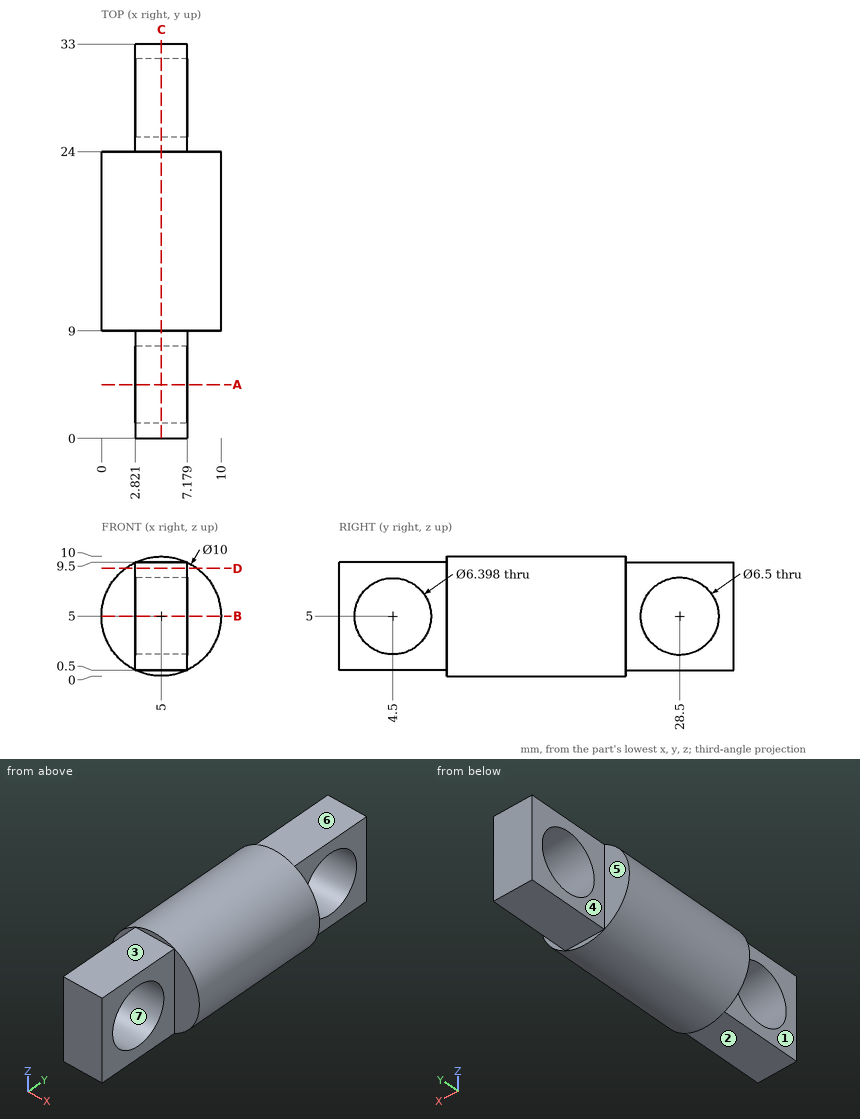
Can you work these out from the drawing? Everything is in mm from the part's minimum corner. A direction names the side the tool comes from. Give positions to 0.01 mm unless a question says otherwise; leave off trailing zeros. Order: outer loops, then holes, each group sorted by start corner. A loop starts at its lowest first (then second) coordinate and runs counter-clockwise, first axis right, second up. Notation, with made-up numbers: M 42.25,-8 L 46.25,-8 A9 cw 46.25,1 Z; hole C 62.5,-4 d4. An arc over 180 degrees is marked long. One line per item, written item: value.
Item 1: If we section it at A-A on y = 4.5: Write out the boundary of the cut face in (x, z).
Verdict:
outline: M 2.82,0.5 L 7.18,0.5 L 7.18,1.8 L 2.82,1.8 Z; M 2.82,8.2 L 7.18,8.2 L 7.18,9.5 L 2.82,9.5 Z
Item 2: For pin 1 (3 mm diameter, centred on x = 7, y = 11.5, fed in from +Z) (1 decimal); pin 2 (2.5 mm diameter, centred on x = 8.5, z = 4.5, fed in from +Y); pin 3 (5 mm diameter, centred on x = 4.5, y = 29.5, fed in from -Z), each with a flat end and sliding along its axis, tell me the tip position at first contact or that it passes through.
Verdict:
pin 1: z = 10
pin 2: y = 24
pin 3: z = 0.5
Item 3: If we mould it in two halves opening along Z, with no side actions, what happens to the marked faces 5, 6 and 7? For each: pulls with the +Z half, pulls with the -Z half, needs draft (parallel to the pull), parting line crosses it, or undercut.
Verdict:
face 5: needs draft
face 6: pulls with the +Z half
face 7: undercut
Item 4: For the marked faces 1, 2, 3 and 4, which set-ups out of +Z, -Z, +X, -X, +Y, -Y let a thin tool reach every point of the face, with its end or its side?
Verdict:
face 1: +Z, -Z, -X, -Y
face 2: -Z, +X, -X, -Y
face 3: +Z, +X, -X, -Y
face 4: +Z, -Z, -X, +Y
Item 5: If we section it at C-C on x = 5: Write out the boundary of the cut face in (y, z), and give its area (3 significant figures).
Verdict:
outline: M 0,0.5 L 9,0.5 L 9,0 L 24,0 L 24,0.5 L 33,0.5 L 33,9.5 L 24,9.5 L 24,10 L 9,10 L 9,9.5 L 0,9.5 Z; hole C 4.5,5 d6.4; hole C 28.5,5 d6.5
area: 247 mm2
Item 6: Please list where these lines run through material, in increasing order: line 1 (Z direction, x = 5.4, y = 4.5); line 2 (Y direction, x = 3.75, z = 2.25) (1 decimal); line 3 (Y direction, x = 7.5, z = 2.75).
Verdict:
line 1: 0.5 to 1.8, 8.2 to 9.5
line 2: 0 to 2.9, 6.1 to 26.8, 30.2 to 33
line 3: 9 to 24
Item 7: If we section it at B-B on z = 5: Write out the boundary of the cut face in (x, y), and give its area (3 significant figures).
Verdict:
outline: M 0,9 L 2.82,9 L 2.82,7.7 L 7.18,7.7 L 7.18,9 L 10,9 L 10,24 L 7.18,24 L 7.18,25.25 L 2.82,25.25 L 2.82,24 L 0,24 Z; M 2.82,0 L 7.18,0 L 7.18,1.3 L 2.82,1.3 Z; M 2.82,31.75 L 7.18,31.75 L 7.18,33 L 2.82,33 Z
area: 172 mm2
Item 8: If we section it at D-D on z = 9: Write out the boundary of the cut face in (x, y).
Verdict:
outline: M 2,9 L 2.82,9 L 2.82,0 L 7.18,0 L 7.18,9 L 8,9 L 8,24 L 7.18,24 L 7.18,33 L 2.82,33 L 2.82,24 L 2,24 Z
